Build history of the part. All positions in model axes, mm. A direction names the side the tool comes from. Round coordinates to 2 decimals unless told otherwise and drop trailing zeros. Order: outer loops, then holes, each group sorted by start corner. A loop starts at its lowest first (then second) coordinate and runs counter-clockwise, first axis right, second up. Notation, with made-up numbers: (87.5, -14.5) -> (146.5, -14.5) arc R12 cw to (146.5, 0.5) -> close; hole circle Ø11 at (30.5, 65). An arc over 180 degrees is marked (long way). Use a Markdown table: item, result. Add a question column.
Item 1: Probe L1, parallel to Z at x = 0, y = 6.65; L2, parallel to Y at x = -1.5, z = 9.5; L3, parallel to Y at x = 0, z = 1.8. List the from-to ranges inside material, lowest first.
Item 2: Slice it at C-C, the plane y = -28. Give the cut face in (x, z), plus the area to 3 significant figures.
Item 3: Slice it at A-A, the plane z = 17.5. Give the cut face in (x, y).
Item 4: Slice it at D-D, the plane y = -34. Give the cut face in (x, z).
Item 5: 3-axis set-ups, long thin cutter, end or side, ignore diameter. For faces 4 (the face through (-1, -36, 15)), 5 (the face through (-6, -29, 15)), 6 (the face through (-2, -33, 5)): which of +Z, -Z, +X, -X, +Y, -Y reach the whole face in a straight line?
Item 6: Two-plate mould, pull along X, no slides. Class faces 1 (the face through (7.4, -27.7, 12.3)), 2 (the face through (1.901, -0.535, -3.232)), 3 (the face through (2, 7.8, 1)): released by +X, released by -X, zero draft, split by the parting line, or undercut.
Item 7: Slice it at B-B, the plane z = 7. Give the cut face in (x, y), plus the area to 3 significant figures.
Item 8: Pin check, flat tips, straight feed: pin 1 (8 mm diameter, centred on x = 9.5, y = -12, fed in from +Z); pin 2 (8 mm diameter, centred on x = 10, y = -10.5, fed in from -Z); pin 3 (3 mm diameter, centred on x = 7, z = 5, fed in from -Y). Stop position of each tip, or through.
from build123d import *
from build123d import SkipClean  # not in build123d's __all__

# Parameters (mm, degrees)
F1_ANGLE  = 180
F2_R      = 13
F3_DEPTH  = 6
F4_R      = 2
F5_DEPTH  = 6
F7_DEPTH  = 2
F8_DEPTH  = 5
F9_DEPTH  = 3
F10_W     = 7.5
F10_H     = 12.1405349095
F11_DEPTH = 2
F12_R     = 2.8
F12_R_2   = 2
F13_DEPTH = 1.8
F14_R     = 3.3
F15_DEPTH = 25
F17_R     = 4.9
F18_DEPTH = 7.3
F19_DEPTH = 25
F20_R     = 7.75
F20_R_2   = 3.3
F21_DEPTH = 25
F23_DEPTH = 20


# Not quite as in the source:
# - after a boolean that leaves OpenCascade's solid faulty, fix() repairs it


with BuildPart() as f1:
    # F0 (on Top) → F1 (revolve)
    with BuildSketch(Plane.XY):
        with BuildLine():
            Line((13, 0), (0, 0))
            Line((0, 0), (0, -43))
            ThreePointArc((0, -43), (9.1923881554, -39.1923881554), (13, -30))
            Line((13, -30), (13, 0))
        make_face()
    revolve(axis=Axis((0, -21.5, 0), (0, 1, 0)), revolution_arc=F1_ANGLE)

    # F2 (on face) → F3 (join)
    with BuildSketch(Plane(origin=(0, 0, 0), x_dir=(-1, 0, 0), z_dir=(0, 1, 0))):
        Circle(F2_R)
    with SkipClean():  # cleaning this boolean's faces spoils the solid; the shape is the same uncleaned
        extrude(amount=F3_DEPTH)

    # F4 (on face) → F5 (cut)
    with BuildSketch(Plane(origin=(0, 6, 0), x_dir=(-1, 0, 0), z_dir=(0, 1, 0))):
        Circle(F4_R)
    extrude(amount=-F5_DEPTH, mode=Mode.SUBTRACT)

    add(f1.part.fix(), mode=Mode.REPLACE)

    # F6 (on face) → F7 (cut)
    with BuildSketch(Plane(origin=(0, 0, 0), x_dir=(-1, 0, 0), z_dir=(0, 1, 0))):
        Polygon((3.75, 2.1650635095), (0, 4.3301270189), (-3.75, 2.1650635095), (-3.75, -2.1650635095), (0, -4.3301270189), (3.75, -2.1650635095), align=None)
    extrude(amount=F7_DEPTH, mode=Mode.SUBTRACT)

    # F8 (cut): a face of the model
    f8_faces = [f1.faces().sort_by_distance(p)[0] for p in [
        (-3.6354356076, 2, 0),
    ]]
    extrude(f8_faces, amount=F8_DEPTH, mode=Mode.SUBTRACT)

    # F9 (cut): a face of the model
    f9_faces = [f1.faces().sort_by_distance(p)[0] for p in [
        (0, 0, -0.8488263632),
    ]]
    extrude(f9_faces, amount=-F9_DEPTH, mode=Mode.SUBTRACT)

    # F10 (on face) → F11 (cut)
    with BuildSketch(Plane.XZ):
        with Locations((0, 8.2353309642)):
            Rectangle(F10_W, F10_H)
    extrude(amount=-F11_DEPTH, mode=Mode.SUBTRACT)

    # F12 (on face) → F13 (join)
    with BuildSketch(Plane(origin=(0, 6, 0), x_dir=(-1, 0, 0), z_dir=(0, 1, 0))):
        Circle(F12_R)
        Circle(F12_R_2, mode=Mode.SUBTRACT)
    extrude(amount=F13_DEPTH)

    # F14 (on face) → F15 (cut)
    with BuildSketch(Plane.XY):
        with Locations((0, -30)):
            Circle(F14_R)
    extrude(amount=-F15_DEPTH, mode=Mode.SUBTRACT)

    # F17 (on face) → F18 (cut)
    with BuildSketch(Plane.XY.offset(-12.5741798937)):
        with Locations((0, -30)):
            Circle(F17_R)
    extrude(amount=F18_DEPTH, mode=Mode.SUBTRACT)

    # F19 (cut): a face of the model
    f19_faces = [f1.faces().sort_by_distance(p)[0] for p in [
        (-4.7614070709, -30, -5.2741798937),
    ]]
    extrude(f19_faces, amount=F19_DEPTH, mode=Mode.SUBTRACT)

    # F20 (on face) → F21 (join)
    with BuildSketch(Plane.XY):
        with Locations((0, -30)):
            Circle(F20_R)
        with Locations((0, -30)):
            Circle(F20_R_2, mode=Mode.SUBTRACT)
    extrude(amount=F21_DEPTH)

    # F22 (on face) → F23 (cut)
    with BuildSketch(Plane.XY.offset(25)):
        with BuildLine():
            ThreePointArc((4.6435439053, -31), (4.7233109971, -30.502825243), (4.75, -30))
            ThreePointArc((4.75, -30), (4.7233109971, -29.497174757), (4.6435439053, -29))
            Line((4.6435439053, -29), (1, -29))
            Line((1, -29), (1, -31))
            Line((1, -31), (4.6435439053, -31))
        make_face()
        with BuildLine():
            ThreePointArc((4.6435439053, -29), (4.7233109971, -29.497174757), (4.75, -30))
            ThreePointArc((4.75, -30), (4.7233109971, -30.502825243), (4.6435439053, -31))
            Line((4.6435439053, -31), (10.7483885819, -31))
            Line((10.7483885819, -31), (10.7483885819, -29))
            Line((10.7483885819, -29), (4.6435439053, -29))
        make_face()
        with BuildLine():
            Line((1, -29), (4.6435439053, -29))
            ThreePointArc((4.6435439053, -29), (3.3587572106, -26.6412427894), (1, -25.3564560947))
            Line((1, -25.3564560947), (1, -29))
        make_face()
        with BuildLine():
            ThreePointArc((1, -34.6435439053), (3.3587572106, -33.3587572106), (4.6435439053, -31))
            Line((4.6435439053, -31), (1, -31))
            Line((1, -31), (1, -34.6435439053))
        make_face()
        with BuildLine():
            Line((1, -29), (1, -25.3564560947))
            ThreePointArc((1, -25.3564560947), (0, -25.25), (-1, -25.3564560947))
            Line((-1, -25.3564560947), (-1, -29))
            Line((-1, -29), (1, -29))
        make_face()
        with BuildLine():
            ThreePointArc((-1, -25.3564560947), (0, -25.25), (1, -25.3564560947))
            Line((1, -25.3564560947), (1, -19.8912940045))
            Line((1, -19.8912940045), (-1, -19.8912940045))
            Line((-1, -19.8912940045), (-1, -25.3564560947))
        make_face()
        with BuildLine():
            Line((1, -40.1087059955), (1, -34.6435439053))
            ThreePointArc((1, -34.6435439053), (0, -34.75), (-1, -34.6435439053))
            Line((-1, -34.6435439053), (-1, -40.1087059955))
            Line((-1, -40.1087059955), (1, -40.1087059955))
        make_face()
        with BuildLine():
            ThreePointArc((-1, -34.6435439053), (0, -34.75), (1, -34.6435439053))
            Line((1, -34.6435439053), (1, -31))
            Line((1, -31), (-1, -31))
            Line((-1, -31), (-1, -34.6435439053))
        make_face()
        with BuildLine():
            Line((-1, -29), (-1, -25.3564560947))
            ThreePointArc((-1, -25.3564560947), (-3.3587572106, -26.6412427894), (-4.6435439053, -29))
            Line((-4.6435439053, -29), (-1, -29))
        make_face()
        with BuildLine():
            Line((-1, -31), (-1, -29))
            Line((-1, -29), (-4.6435439053, -29))
            ThreePointArc((-4.6435439053, -29), (-4.75, -30), (-4.6435439053, -31))
            Line((-4.6435439053, -31), (-1, -31))
        make_face()
        with BuildLine():
            ThreePointArc((-4.6435439053, -31), (-3.3587572106, -33.3587572106), (-1, -34.6435439053))
            Line((-1, -34.6435439053), (-1, -31))
            Line((-1, -31), (-4.6435439053, -31))
        make_face()
        with BuildLine():
            ThreePointArc((-4.6435439053, -31), (-4.75, -30), (-4.6435439053, -29))
            Line((-4.6435439053, -29), (-10.7483885819, -29))
            Line((-10.7483885819, -29), (-10.7483885819, -31))
            Line((-10.7483885819, -31), (-4.6435439053, -31))
        make_face()
    extrude(amount=-F23_DEPTH, mode=Mode.SUBTRACT)


solid = f1.part
Check sheet entries:
| question | item | result |
|---|---|---|
| 1 | L1 | -2.8 to -2, 2 to 2.8 |
| 1 | L2 | -37.6 to -34.51, -25.49 to -22.4, 2 to 6 |
| 1 | L3 | -37.75 to -33.3, -26.7 to -22.25 |
| 2 | outline | (-13, 0) arc R13 ccw to (-4.47, -12.21) -> (-4.47, -5.27) -> (-2.62, -5.27) -> (-2.62, 5) -> (-4.31, 5) -> (-4.31, 25) -> (-7.49, 25) -> (-7.49, 0) -> close; (2.62, -5.27) -> (4.47, -5.27) -> (4.47, -12.21) arc R13 ccw to (13, 0) -> (7.49, 0) -> (7.49, 25) -> (4.31, 25) -> (4.31, 5) -> (2.62, 5) -> close |
| 2 | area | 347 mm2 |
| 3 | outline | (-7.69, -31) arc R7.75 ccw to (-1, -37.69) -> (-1, -34.64) arc R4.75 cw to (-4.64, -31) -> close; (-7.69, -29) -> (-4.64, -29) arc R4.75 cw to (-1, -25.36) -> (-1, -22.31) arc R7.75 ccw to start; (1, -37.69) arc R7.75 ccw to (7.69, -31) -> (4.64, -31) arc R4.75 cw to (1, -34.64) -> close; (1, -25.36) arc R4.75 cw to (4.64, -29) -> (7.69, -29) arc R7.75 ccw to (1, -22.31) -> close |
| 4 | outline | (-12.37, 0) arc R12.37 ccw to (-2.83, -12.04) -> (-2.83, -5.27) -> (2.83, -5.27) -> (2.83, -12.04) arc R12.37 ccw to (12.37, 0) -> (6.64, 0) -> (6.64, 25) -> (2.56, 25) -> (2.56, 5) -> (-2.56, 5) -> (-2.56, 25) -> (-6.64, 25) -> (-6.64, 0) -> close |
| 5 | face 4 | +Z, -Y |
| 5 | face 5 | +Z, +X, -X |
| 5 | face 6 | +Z |
| 6 | face 1 | split by the parting line |
| 6 | face 2 | undercut |
| 6 | face 3 | zero draft |
| 7 | outline | (-10.95, 0) -> (-3.75, 0) -> (-3.75, 2) -> (3.75, 2) -> (3.75, 0) -> (10.95, 0) -> (10.95, 6) -> (-10.95, 6) -> close; (-7.69, -31) arc R7.75 ccw to (-1, -37.69) -> (-1, -34.64) arc R4.75 cw to (-4.64, -31) -> close; (-7.69, -29) -> (-4.64, -29) arc R4.75 cw to (-1, -25.36) -> (-1, -22.31) arc R7.75 ccw to start; (1, -37.69) arc R7.75 ccw to (7.69, -31) -> (4.64, -31) arc R4.75 cw to (1, -34.64) -> close; (1, -25.36) arc R4.75 cw to (4.64, -29) -> (7.69, -29) arc R7.75 ccw to (1, -22.31) -> close |
| 7 | area | 210 mm2 |
| 8 | pin 1 | z = 0 |
| 8 | pin 2 | z = -11.53 |
| 8 | pin 3 | y = -35.46 |
